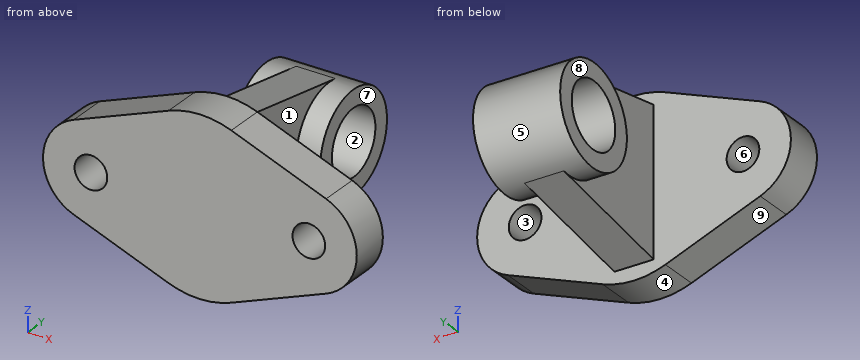
Autodesk Inventor part; units mm, degrees
ref_plane "YZ Plane" through (0, 0, 0) normal (1, 0, 0) x (0, 1, 0)
ref_plane "XZ Plane" through (0, 0, 0) normal (0, 1, 0) x (-1, 0, 0)
ref_plane "XY Plane" through (0, 0, 0) normal (0, 0, 1) x (1, 0, 0)
sketch "Sketch1" plane through (0, 0, 0) normal (0, 1, 0) x (-1, 0, 0)
  line L0 (50, 0) -> (-50, 0) construction
  line L1 (50, 22) -> (-50, 22)
  line L2 (-50, -22) -> (50, -22)
  arc A0 (50, -22) -> (50, 22) centre (50, 0) ccw
  arc A1 (-50, 22) -> (-50, -22) centre (-50, 0) ccw
  circle A2 centre (50, 0) radius 7.5
  circle A3 centre (-50, 0) radius 7.5
  line L3 (57.92, 20.525) -> (14.4, 37.3181)
  line L4 (-14.4, 37.3181) -> (-57.92, 20.525)
  line L5 (0, 0) -> (0, 42.8746) construction
  arc A4 (14.4, 37.3181) -> (-14.4, 37.3181) centre (0, 0) ccw
  line L6 (57.92, -20.525) -> (14.4, -37.3181)
  line L7 (-14.4, -37.3181) -> (-57.92, -20.525)
  line L8 (0, 0) -> (0, -42.8746) construction
  arc A5 (-14.4, -37.3181) -> (14.4, -37.3181) centre (0, 0) ccw
  point P0 (-57.92, -20.525)
  dimension "d0" = 100
  dimension "d1" = 40
  dimension "d2" = 15
  dimension "d3" = 22
extrude "Extrusion1" add sketch "Sketch1" along normal blind 18
sketch "Sketch2" plane through (0, 0, 0) normal (1, 0, 0) x (0, 1, 0)
  line L0 (0, 0) -> (76, 0) construction
  circle A0 centre (76, 0) radius 23
  circle A1 centre (76, 0) radius 15
  line L1 (18, -20.525) -> (18, -37.3181) construction
  line L2 (18, -37.3181) -> (18, -37.3181) construction
  line L3 (18, -37.3181) -> (18, -20.525) construction
  line L4 (18, -20.525) -> (18, 20.525) construction
  line L5 (18, 20.525) -> (18, 37.3181) construction
  line L6 (18, 37.3181) -> (18, 37.3181) construction
  line L7 (18, 37.3181) -> (18, 20.525) construction
  line L8 (18, 20.525) -> (18, -20.525) construction
  line L9 (18, 7.5) -> (18, -7.5) construction
  line L10 (18, 7.5) -> (18, -7.5) construction
  line L11 (79.9649, -22.6557) -> (18, -33.5)
  line L12 (79.9649, 22.6557) -> (18, 33.5)
  line L13 (18, -33.5) -> (18, 33.5)
  point P0 (79.9649, 22.6557)
  point P1 (18, 0)
  dimension "d8" = 46
  dimension "d7" = 67
  dimension "d9" = 30
  dimension "d14" = 116
extrude "Extrusion2" add sketch "Sketch2" along normal mid plane 18
extrude "Extrusion3" add sketch "Sketch2" along normal mid plane 40 contours A0
properties part number "ShaftSupport"
Work out the finished part from the listing and answer in its coordinate system (mm). Face numbers are marked on the shaded views. A direction names the side the tool comes from. Round coordinates to 2 decimals unless told otherwise and drop trailing zeros. Loops run counter-clockwise (first coordinate to the right, second up) from the corner with the lowest first, then second, coordinate; pieces in that order, holes last. Notation, with made-up numbers: M 47.25,62.25 L 80.25,62.25 A26 cw 80.25,89.25 Z; hole C 34,56.5 d1. An arc over 180 degrees is marked long. One line per question, with ' | ' between items. Start each with the question number.
(1) A cutting plane is placed at D-D on y = 76. Write down the section's boundary in (x, z).
(2) A cutting plane is placed at A-A on z = 0. Write down the section's boundary in (x, y).
(3) For a pull along X with two mould halves and no side action, classify the marked faces 1, 2, 3 and 4 as released by +X, released by -X, zero draft, split by the parting line, or undercut.
(4) A cutting plane is placed at B-B on y = 12. Write down the section's boundary in (x, z) (3 decimals), plus the area to 3 significant figures.
(5) Find the intervals of material crossed by line 1 (X direction, y = 63, z = 10.5); line 2 (Z direction, x = 50, y = 9.75); line 3 (Y direction, x = 39.5, z = -26), in increasing order.
(6) A tool of negligible diameter and unlimited length cuts with its end or side. For the marked faces 5, 6, 7, 8 and 9, from which of +Z, -Z, +X, -X, +Y, -Y can it reach the whole face along a straight path? Write none if from no direction.
(7) Flat-ended cylindrical pins translate along their axes: pin 1 Ø5 at (x, z) = (-41, 28) entering from +Y; pin 2 Ø1 at (y, z) = (55, -16) entering from -X; pin 3 Ø9 at (x, z) = (50, 0) entering from -Y; pin 4 Ø6 at (y, z) = (69.5, 13) entering from -X. Find the tip coordinate at first contact, or state that the pin passes through.
(8) A cutting plane is placed at C-C on x = -50. Write down the section's boundary in (y, z).
Geometry check:
1) outline: M -20,-23 L -9,-23 L -9,-23.35 L 9,-23.35 L 9,-23 L 20,-23 L 20,-15 L -20,-15 Z; M -20,15 L 20,15 L 20,23 L 9,23 L 9,23.35 L -9,23.35 L -9,23 L -20,23 Z
2) outline: M -72,0 L -57.5,0 L -57.5,18 L -72,18 Z; M -42.5,0 L 42.5,0 L 42.5,18 L 9,18 L 9,53 L 20,53 L 20,61 L -20,61 L -20,53 L -9,53 L -9,18 L -42.5,18 Z; M -20,91 L 20,91 L 20,99 L -20,99 Z; M 57.5,0 L 72,0 L 72,18 L 57.5,18 Z
3) face 1: released by +X | face 2: zero draft | face 3: undercut | face 4: split by the parting line
4) outline: M -57.92,-20.525 L -14.4,-37.318 A40 ccw 14.4,-37.318 L 57.92,-20.525 A22 ccw 57.92,20.525 L 14.4,37.318 A40 ccw -14.4,37.318 L -57.92,20.525 A22 ccw Z; hole C -50,0 d15; hole C 50,0 d15 | area: 7,770 mm²
5) line 1: x = -20 to 20 | line 2: z = -23.58 to -7.5, 7.5 to 23.58 | line 3: y = 0 to 18
6) face 5: none | face 6: +Y, -Y | face 7: +Z, -Z, +X, +Y | face 8: +Z, -Z, -X, +Y | face 9: -Z, -X, +Y, -Y
7) pin 1: stops at y = 18 | pin 2: stops at x = -9 | pin 3: passes through | pin 4: stops at x = -20
8) outline: M 0,-23.58 L 18,-23.58 L 18,-7.5 L 0,-7.5 Z; M 0,7.5 L 18,7.5 L 18,23.58 L 0,23.58 Z
